The listing builds one solid part. Answer for the finished solid, in the listing's coordinates (mm). Face numbers are marked on the shaded views. A direction names the side the tool comes from. Coordinates: 2 decimals unless noted, no trailing zeros. Write each loop counter-clockwise with the first axis right and the second up, starting at its lowest first coordinate (ties: lowest second). Pieces come first, ordered by that corner, then holes. Notation, with made-up numbers: M 79.25,58.25 L 99.25,58.25 A15 ccw 99.25,82.25 Z; hole C 31.5,21.5 d8. An arc over 180 degrees is marked long. Put each result on its own line as item: value. Start each with the question number.
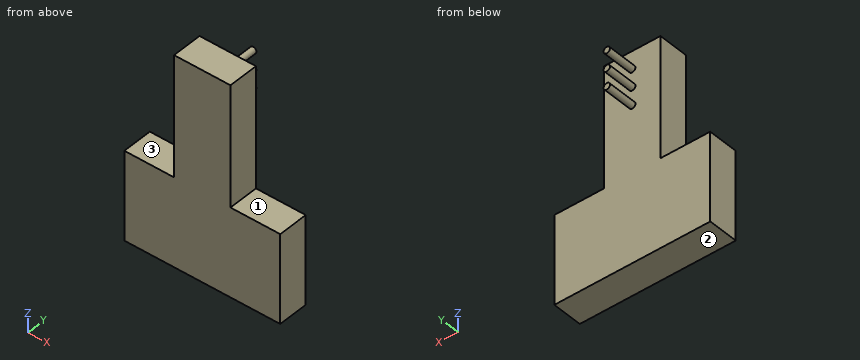
```python
from build123d import *

# Parameters (mm, degrees)
BOSS_EXTRUDE1_DEPTH = 30
SKETCH2_R           = 3.175
BOSS_EXTRUDE2_DEPTH = 30


with BuildPart() as part:
    # Sketch1 → Boss-Extrude1 (new body)
    with BuildSketch(Plane(origin=(0, 0, 0), x_dir=(1, 0, 0), z_dir=(0, 1, 0))):
        Polygon((28, 0), (77.5, 0), (77.5, 88.2), (-77.5, 88.2), (-77.5, 0), (-28, 0), (-28, -120), (28, -120), align=None)
    extrude(amount=-BOSS_EXTRUDE1_DEPTH)

    # Sketch2 → Boss-Extrude2 (add)
    with BuildSketch(Plane(origin=(0, 0, 0), x_dir=(1, 0, 0), z_dir=(0, 1, 0))):
        with Locations(Location((0, -84.44, 0), (0, 0, 90))):
            Circle(SKETCH2_R)
        with Locations(Location((0, -66.66, 0), (0, 0, 90))):
            Circle(SKETCH2_R)
        with Locations(Location((0, -102.22, 0), (0, 0, 90))):
            Circle(SKETCH2_R)
    extrude(amount=BOSS_EXTRUDE2_DEPTH)


solid = part.part
```
1) A cutting plane is placed at B-B on x = 0. Write down the section's boundary in (y, z) (3 decimals), then the cut area to 3 significant figures.
2) Straight lines are drawn through the part: probe 1 along X at (y, z) = (-11, 1); probe 2 along Z at (x, y) = (34.5, -13); probe 3 along Y at (x, z) = (6, 43). For each, find the intervals that lie inside material, in ascending order.
3) A cutting plane is placed at D-D on z = 66.66. Write down the section's boundary in (x, y) (3 decimals), then the cut area to 3 significant figures.
4) For the marked faces 1, 2 and 3, determine the directions among +Z, -Z, +X, -X, +Y, -Y from which every point of the face is accessible in a straight line to the end or side of a thin tool.
5) A cutting plane is placed at C-C on y = 13. Write down the section's boundary in (x, z) (3 decimals).
6) A cutting plane is placed at A-A on y = -15.5. Write down the section's boundary in (x, z).
7) Given pin 1 Ø10 at (x, z) = (47.5, -64.5) entering from +Y; pin 2 Ø12 at (y, z) = (2.5, 20.5) entering from +X; pin 3 Ø9 at (x, y) = (63.5, -13) entering from +Z, each flat-ended and moving along its own axis, determine where each tip first touches the part or whether it passes through.
Answers follow:
1. outline: M -30,-88.2 L 0,-88.2 L 0,63.485 L 30,63.485 L 30,69.835 L 0,69.835 L 0,81.265 L 30,81.265 L 30,87.615 L 0,87.615 L 0,99.045 L 30,99.045 L 30,105.395 L 0,105.395 L 0,120 L -30,120 Z
1. area: 6,820 mm²
2. probe 1: x = -28 to 28
2. probe 2: z = -88.2 to 0
2. probe 3: y = -30 to 0
3. outline: M -28,-30 L 28,-30 L 28,0 L 3.175,0 L 3.175,30 L -3.175,30 L -3.175,0 L -28,0 Z
3. area: 1,870 mm²
4. face 1: +Z, +X, +Y, -Y
4. face 2: -Z, +X, -X, +Y, -Y
4. face 3: +Z, -X, +Y, -Y
5. outline: C 0,66.66 d6.35; C 0,84.44 d6.35; C 0,102.22 d6.35
6. outline: M -77.5,-88.2 L 77.5,-88.2 L 77.5,0 L 28,0 L 28,120 L -28,120 L -28,0 L -77.5,0 Z
7. pin 1: stops at y = 0
7. pin 2: stops at x = 28
7. pin 3: stops at z = 0
